CAD build for the part. Positions are in the model's coordinates, mm. Face numbers are marked on the shaded views. A direction names the side the tool comes from. Give positions to 0.01 mm unless a question says otherwise; leave off trailing zeros. Order: outer loops, then holes, each group sorted by start corner. A loop starts at its lowest first (then second) coordinate and runs counter-clockwise, first axis right, second up.
from build123d import *

# Parameters (mm, degrees)
BOSS_EXTRUDE1_DEPTH        = 31.75
FILLET1_R                  = 6.35
SHELL1_T                   = -3.175
FILLET2_R                  = 1.27
CHAMFER1_SIZE              = 1.905
F_9_0_196_DIAMETER_HOLE1_D = 4.9784
F_9_0_196_DIAMETER_HOLE2_D = 4.9784
F_9_0_196_DIAMETER_HOLE3_D = 4.9784


with BuildPart() as part:
    # Sketch1 → Boss-Extrude1 (new body)
    with BuildSketch(Plane(origin=(0, 0, 0), x_dir=(1, 0, 0), z_dir=(0, 1, 0))):
        Polygon((-57.15, 0), (0, 0), (0, -38.1), (31.75, -38.1), (31.75, -50.8), (-12.7, -50.8), (-12.7, -12.7), (-57.15, -12.7), align=None)
    extrude(amount=BOSS_EXTRUDE1_DEPTH)

    # Fillet1
    fillet1_edges = [part.edges().sort_by_distance(p)[0] for p in [
        (0, 15.875, 0),
        (0, 15.875, 38.1),
        (-12.7, 15.875, 50.8),
        (-12.7, 15.875, 12.7),
    ]]
    fillet(fillet1_edges, radius=FILLET1_R)

    # Shell1
    shell1_openings = [part.faces().sort_by_distance(p)[0] for p in [
        (-8.466666667, 31.75, 25.4),
        (31.75, 15.875, 44.45),
        (-57.15, 15.875, 6.35),
    ]]
    offset(amount=SHELL1_T, openings=shell1_openings, kind=Kind.INTERSECTION)

    # Fillet2
    fillet2_edges = [part.edges().sort_by_distance(p)[0] for p in [
        (-38.1, 0, 12.7),
        (12.7, 0, 50.8),
        (-31.75, 0, 0),
        (0, 0, 19.05),
        (-12.7, 0, 31.75),
        (-1.859871939, 0, 1.859871939),
        (-10.840128061, 0, 48.940128061),
        (-14.559871939, 0, 14.559871939),
        (1.859871939, 0, 36.240128061),
        (19.05, 0, 38.1),
    ]]
    fillet(fillet2_edges, radius=FILLET2_R)

    # Chamfer1
    chamfer1_edges = [part.edges().sort_by_distance(p)[0] for p in [
        (-9.525, 31.75, 31.75),
        (-8.59506403, 31.75, 46.69506403),
        (12.7, 31.75, 47.625),
        (19.05, 31.75, 41.275),
        (-0.385192091, 31.75, 38.485192091),
        (-3.175, 31.75, 19.05),
        (-4.10493597, 31.75, 4.10493597),
        (-31.75, 31.75, 3.175),
        (-38.1, 31.75, 9.525),
        (-12.314807909, 31.75, 12.314807909),
    ]]
    chamfer(chamfer1_edges, length=CHAMFER1_SIZE)

    # #9 (0.196) Diameter Hole1 (through all)
    with Locations(Plane.ZY.offset(12.7)):
        with Locations((25.4, 15.875)):
            Hole(F_9_0_196_DIAMETER_HOLE1_D / 2)

    # #9 (0.196) Diameter Hole2 (through all)
    with Locations(Plane(origin=(0, 0, 0), x_dir=(-1, 0, 0), z_dir=(0, 0, -1))):
        with Locations((44.45, 16.51)):
            Hole(F_9_0_196_DIAMETER_HOLE2_D / 2)

    # #9 (0.196) Diameter Hole3 (through all)
    with Locations(Plane.XY.offset(50.8)):
        with Locations((25.4, 16.51)):
            Hole(F_9_0_196_DIAMETER_HOLE3_D / 2)


solid = part.part
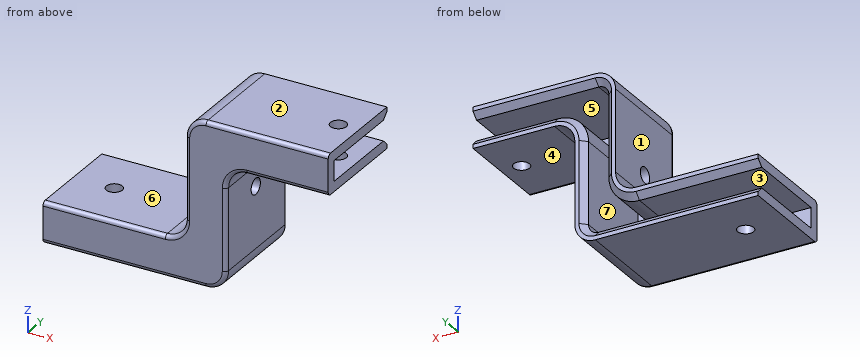
1. 3-axis set-ups, long thin cutter, end or side, ignore diameter. For the marked faces 4, 5, 6 and 7: which of +Z, -Z, +X, -X, +Y, -Y reach the whole face in a straight line?
2. Wall check: line 1 (Z direction, x = -45, y = 23) (3 decimals); line 2 (Y direction, x = -1.15, z = 25.4); line 3 (Z direction, x = 12, y = 17) (3 decimals). Give the ranges that are in metal, low to high.
3. Pin check, flat tips, straight feed: P1, Ø5.5, axis at x = 25.4, y = 16.51, coming from the -Z side; P2, Ø2, axis at y = 10, z = 19.5, coming from the +X side; P3, Ø9, axis at x = -39.5, y = 17.5, coming from the +Z side; P4, Ø3, axis at x = -44.45, y = 16.51, coming from the +Z side. Stop position of each tip, or through.
4. Saw through at C-C on y = 10. Give the cut face in (x, z) (3 decimals).
5. Saw through at D-D on x = -24. Give the cut face in (y, z) (3 decimals).
6. Saw through at B-B on z = 25.4. Give the cut face in (x, y) (3 decimals).
7. Mould opens along Z. For the marked faces 1, 2 and 3 say: released by +Z, released by -Z, zero draft, split by the parting line, or undercut.
8. Saw through at A-A on x = -44.45. Give the cut face in (y, z) (3 decimals), plus the area to 3 significant figures.
Reported:
1. face 4: -Z, +X, +Y, -Y
1. face 5: +X, +Y
1. face 6: +Z, -X, +Y, -Y
1. face 7: +Y
2. line 1: z = 0 to 3.175, 9.525 to 12.7
2. line 2: y = 0.01 to 13.39, 18.36 to 31.75
2. line 3: z = 38.1 to 41.275, 47.625 to 50.8
3. P1: stops at z = 38.1
3. P2: stops at x = 0
3. P3: stops at z = 12.7
3. P4: passes through
4. outline: (-57.15, 0) - (-6.35, 0) arc R6.35 ccw to (0, 6.35) - (0, 31.75) arc R6.35 cw to (6.35, 38.1) - (31.75, 38.1) - (31.75, 41.275) - (6.35, 41.275) arc R9.525 ccw to (-3.175, 31.75) - (-3.175, 6.35) arc R3.175 cw to (-6.35, 3.175) - (-57.15, 3.175) - close; (-57.15, 9.525) - (-19.05, 9.525) arc R9.525 ccw to (-9.525, 19.05) - (-9.525, 44.45) arc R3.175 cw to (-6.35, 47.625) - (31.75, 47.625) - (31.75, 50.8) - (-6.35, 50.8) arc R6.35 ccw to (-12.7, 44.45) - (-12.7, 19.05) arc R6.35 cw to (-19.05, 12.7) - (-57.15, 12.7) - close
5. outline: (0, 1.27) arc R1.27 ccw to (1.27, 0) - (31.75, 0) - (31.75, 1.27) - (29.845, 3.175) - (3.175, 3.175) - (3.175, 9.525) - (29.845, 9.525) - (31.75, 11.43) - (31.75, 12.7) - (1.27, 12.7) arc R1.27 ccw to (0, 11.43) - close
6. outline: (-12.7, 1.27) arc R1.27 ccw to (-11.43, 0) - (-1.27, 0) arc R1.27 ccw to (0, 1.27) - (0, 13.386) - (-3.175, 13.386) - (-3.175, 3.175) - (-9.525, 3.175) - (-9.525, 13.386) - (-12.7, 13.386) - close; (-12.7, 18.364) - (-9.525, 18.364) - (-9.525, 29.845) - (-11.43, 31.75) - (-12.7, 31.75) - close; (-3.175, 18.364) - (0, 18.364) - (0, 31.75) - (-1.27, 31.75) - (-3.175, 29.845) - close
7. face 1: zero draft
7. face 2: released by +Z
7. face 3: undercut
8. outline: (0, 1.27) arc R1.27 ccw to (1.27, 0) - (14.021, 0) - (14.021, 3.175) - (3.175, 3.175) - (3.175, 9.525) - (14.021, 9.525) - (14.021, 12.7) - (1.27, 12.7) arc R1.27 ccw to (0, 11.43) - close; (18.999, 0) - (31.75, 0) - (31.75, 1.27) - (29.845, 3.175) - (18.999, 3.175) - close; (18.999, 9.525) - (29.845, 9.525) - (31.75, 11.43) - (31.75, 12.7) - (18.999, 12.7) - close
8. area: 186 mm2
